Could you check a few things on this model? Use its own coordinates, in mm. Face numbers are marked on the shaded views. Round coordinates to 2 decimals unless told otherwise and drop trailing zeros. Write each loop counter-clockwise with the first axis right and the second up, starting at its lowest first coordinate (ties: lowest second). Pieces come first, ordered by that corner, then holes. Notation, with made-up numbers: (41.25, 19.5) -> (65.25, 19.5) arc R27 cw to (65.25, 58.5) -> close; hole circle Ø11 at (6.5, 79). An arc over 180 degrees is marked (long way). Return JSON: item names as keys, results as strings.
from build123d import *

# Parameters (mm, degrees)
SKETCH_1_W      = 140
SKETCH_1_H      = 116
PAD_DEPTH       = 5
SKETCH_W        = 140
SKETCH_H        = 15
PAD001_DEPTH    = 5
SKETCH001_W     = 131
SKETCH001_H     = 5
PAD002_DEPTH    = 5
SKETCH002_W     = 9.2
SKETCH002_H     = 9.2
POCKET_DEPTH    = 5
SKETCH003_W     = 102.8
SKETCH003_H     = 2
PAD003_DEPTH    = 51
SKETCH004_W     = 2
SKETCH004_H     = 121.8
PAD004_DEPTH    = 51
PAD005_DEPTH    = 53
SKETCH006_W     = 15
SKETCH006_H     = 41
POCKET001_DEPTH = 2
SKETCH007_W     = 9.2
SKETCH007_H     = 5
PAD006_DEPTH    = 9.2
SKETCH008_R     = 1.6
POCKET002_DEPTH = 5
SKETCH009_W     = 33
SKETCH009_H     = 2
PAD007_DEPTH    = 51
SKETCH010_W     = 108.1
SKETCH010_H     = 2.08
POCKET003_DEPTH = 11
SKETCH011_W     = 122.1
SKETCH011_H     = 2.08
POCKET004_DEPTH = 11
CHAMFER_SIZE    = 2
PAD008_DEPTH    = 51
CHAMFER001_SIZE = 2


with BuildPart() as part:
    # Sketch_1 → Pad (new body)
    with BuildSketch(Plane.XY):
        with Locations((-70, 58)):
            Rectangle(SKETCH_1_W, SKETCH_1_H)
    extrude(amount=PAD_DEPTH)

    # Sketch → Pad001 (join)
    with BuildSketch(Plane.XY):
        with Locations((-70, -7.5)):
            Rectangle(SKETCH_W, SKETCH_H)
    extrude(amount=PAD001_DEPTH)

    # Sketch001 (on Face9 of Pad001) → Pad002 (join)
    with BuildSketch(Plane.YZ):
        with Locations((50.5, 2.5)):
            Rectangle(SKETCH001_W, SKETCH001_H)
    extrude(amount=PAD002_DEPTH)

    # Sketch002 (on Face11 of Pad002) → Pocket (cut)
    with BuildSketch(Plane.XY.offset(5)):
        with Locations((0.4, -10.4)):
            Rectangle(SKETCH002_W, SKETCH002_H)
    extrude(amount=-POCKET_DEPTH, mode=Mode.SUBTRACT)

    # Sketch003 (on Face7 of Pocket) → Pad003 (join)
    with BuildSketch(Plane(origin=(0, 0, 0), x_dir=(1, 0, 0), z_dir=(0, 0, -1))):
        with Locations((-55.6, 14)):
            Rectangle(SKETCH003_W, SKETCH003_H)
    extrude(amount=PAD003_DEPTH)

    # Sketch004 (on Face10 of Pad003) → Pad004 (join)
    with BuildSketch(Plane(origin=(0, 0, 0), x_dir=(1, 0, 0), z_dir=(0, 0, -1))):
        with Locations((4, -55.1)):
            Rectangle(SKETCH004_W, SKETCH004_H)
    extrude(amount=PAD004_DEPTH)

    # Sketch005 (on Face7 of Pad004) → Pad005 (join)
    with BuildSketch(Plane(origin=(0, 0, 0), x_dir=(1, 0, 0), z_dir=(0, 0, -1))):
        Polygon((-4.2, 13), (-6.2, 13), (-6.2, 3.8), (3, 3.8), (3, 5.8), (-4.2, 5.8), align=None)
    extrude(amount=PAD005_DEPTH)

    # Sketch006 (on Face12 of Pad005) → Pocket001 (cut)
    with BuildSketch(Plane.XZ.offset(15)):
        with Locations((-23.5, -50.5)):
            Rectangle(SKETCH006_W, SKETCH006_H)
        with Locations((-43.5, -50.5)):
            Rectangle(SKETCH006_W, SKETCH006_H)
        with Locations((-63.5, -50.5)):
            Rectangle(SKETCH006_W, SKETCH006_H)
        with Locations((-83.5, -50.5)):
            Rectangle(SKETCH006_W, SKETCH006_H)
    extrude(amount=-POCKET001_DEPTH, mode=Mode.SUBTRACT)

    # Sketch007 (on Face44 of Pocket001) → Pad006 (join)
    with BuildSketch(Plane.XZ.offset(5.8)):
        with Locations((0.4, -48.5)):
            Rectangle(SKETCH007_W, SKETCH007_H)
    extrude(amount=PAD006_DEPTH)

    # Sketch008 (on Face50 of Pad006) → Pocket002 (cut)
    with BuildSketch(Plane.XY.offset(-46)):
        with Locations((-0.6, -9.4)):
            Circle(SKETCH008_R)
    extrude(amount=-POCKET002_DEPTH, mode=Mode.SUBTRACT)

    # Sketch009 (on Face7 of Pocket002) → Pad007 (join)
    with BuildSketch(Plane(origin=(0, 0, 0), x_dir=(1, 0, 0), z_dir=(0, 0, -1))):
        with Locations((-123.5, 14)):
            Rectangle(SKETCH009_W, SKETCH009_H)
    extrude(amount=PAD007_DEPTH)

    # Sketch010 (on Face1 of Pad007) → Pocket003 (cut)
    with BuildSketch(Plane(origin=(-140, 0, 0), x_dir=(0, -1, 0), z_dir=(-1, 0, 0))):
        with Locations((-41, 2.54)):
            Rectangle(SKETCH010_W, SKETCH010_H)
    extrude(amount=-POCKET003_DEPTH, mode=Mode.SUBTRACT)

    # Sketch011 (on Face3 of Pocket003) → Pocket004 (cut)
    with BuildSketch(Plane(origin=(0, 116, 0), x_dir=(-1, 0, 0), z_dir=(0, 1, 0))):
        with Locations((58, 2.54)):
            Rectangle(SKETCH011_W, SKETCH011_H)
    extrude(amount=-POCKET004_DEPTH, mode=Mode.SUBTRACT)

    # Chamfer
    chamfer_edges = [part.edges().sort_by_distance(p)[0] for p in [
        (-72.1, -15, 5),
        (-4.2, -10.4, 5),
        (-2.1, -5.8, 5),
        (2.5, -5.8, 5),
        (5, 55.1, 5),
    ]]
    chamfer(chamfer_edges, length=CHAMFER_SIZE)

    # Sketch012 (on Face23 of Chamfer) → Pad008 (join)
    with BuildSketch(Plane(origin=(0, 0, 0), x_dir=(1, 0, 0), z_dir=(0, 0, -1))):
        Polygon((2, -114), (2, -117.5), (3, -117.5), (3, -114), (3, -113), align=None)
    extrude(amount=PAD008_DEPTH)

    # Chamfer001
    chamfer001_edges = [part.edges().sort_by_distance(p)[0] for p in [
        (-91, -14, -30),
        (-76, -14, -30),
        (-71, -14, -30),
        (-56, -14, -30),
        (-51, -14, -30),
        (-36, -14, -30),
        (-31, -14, -30),
        (-16, -14, -30),
    ]]
    chamfer(chamfer001_edges, length=CHAMFER001_SIZE)


solid = part.part
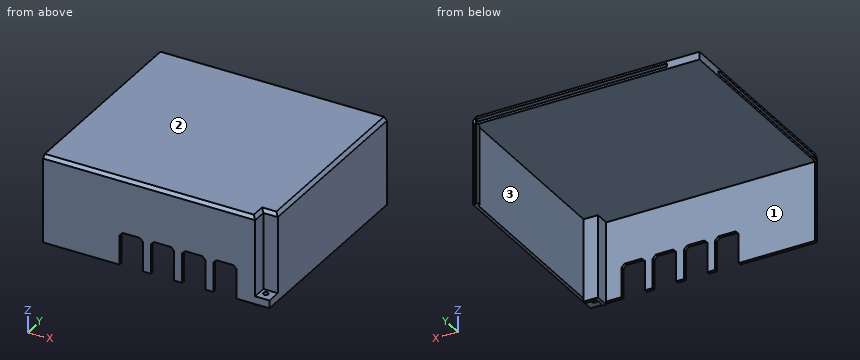
1) I want a section at A-A, the plane z = -43. Count the separate pieces of the cut face and the enclosed holes in it, and give its area (3 significant figures).
Return value:
{"separate pieces": "5", "enclosed holes": "0", "area": "432 mm²"}
2) Will these pins go through, and if not, where does the flat tip stop? pin 1 Ø1.1 at (x, y) = (2.5, 117) entering from +Z; pin 2 Ø2 at (y, z) = (104, -28) entering from -X; pin 3 Ø1 at (y, z) = (-14, -41) entering from +X.
Return value:
{"pin 1": "z = 0", "pin 2": "x = 3", "pin 3": "x = -4.2"}
3) I want a section at B-B, the plane z = -23. Please give me the cut outline in (x, y), and give its area (3 significant figures).
Return value:
{"outline": "(-140, -15) -> (-4.2, -15) -> (-4.2, -5.8) -> (5, -5.8) -> (5, 116) -> (3, 116) -> (3, 117.5) -> (2, 117.5) -> (2, 114) -> (3, 113) -> (3, -3.8) -> (-6.2, -3.8) -> (-6.2, -13) -> (-140, -13) -> close", "area": "552 mm²"}
4) Thinking about a two-plate mould opening in Y: for the marked faces 1, 2 and 3, which applies, pulls with the +Y half, pulls with the -Y half, needs draft (parallel to the pull), parting line crosses it, or undercut?
Return value:
{"face 1": "pulls with the +Y half", "face 2": "needs draft", "face 3": "undercut"}
5) I want a section at C-C, the plane y = 53.5. Please give me the cut outline in (x, z), and give its area (3 significant figures).
Return value:
{"outline": "(-140, 0) -> (3, 0) -> (3, -51) -> (5, -51) -> (5, 3) -> (3, 5) -> (-140, 5) -> (-140, 3.58) -> (-129, 3.58) -> (-129, 1.5) -> (-140, 1.5) -> close", "area": "802 mm²"}
6) If I drill on probe 1 along Y at (x, z) = (-0.6, -49.8); probe 2 along Z at (x, y) = (-38.5, 111.5); probe 3 along Z at (x, y) = (-80, 99.5), over which ranges is the centre line in solid material (lowest first)? Write a range as [from, to].
Return value:
{"probe 1": "[-15, -11], [-7.8, -3.8]", "probe 2": "[0, 1.5], [3.58, 5]", "probe 3": "[0, 5]"}
7) I want a section at D-D, the plane x = -95. Please give me the cut outline in (y, z), and give its area (3 significant figures).
Return value:
{"outline": "(-15, -51) -> (-13, -51) -> (-13, 0) -> (116, 0) -> (116, 1.5) -> (105, 1.5) -> (105, 3.58) -> (116, 3.58) -> (116, 5) -> (-13, 5) -> (-15, 3) -> close", "area": "732 mm²"}
